```python
from build123d import *

# Parameters (mm, degrees)
SKETCH_1_W      = 10
SKETCH_1_H      = 30
SKETCH_1_R      = 1.5
EXTRUDE_1_DEPTH = 2
FILLET_1_R      = 1


with BuildPart() as part:
    # 草图1 → 凸台-拉伸1 (new body)
    with BuildSketch(Plane.XY):
        with Locations((1.642083631, -16.90903272)):
            Rectangle(SKETCH_1_W, SKETCH_1_H)
        with Locations((1.642083631, -6.90903272)):
            Circle(SKETCH_1_R, mode=Mode.SUBTRACT)
        with Locations((1.642083631, -16.90903272)):
            Circle(SKETCH_1_R, mode=Mode.SUBTRACT)
        with Locations((1.642083631, -26.90903272)):
            Circle(SKETCH_1_R, mode=Mode.SUBTRACT)
    extrude(amount=EXTRUDE_1_DEPTH)

    # 圆角1
    fillet_1_edges = [part.edges().sort_by_distance(p)[0] for p in [
        (-3.357916369, -1.90903272, 1),
        (6.642083631, -1.90903272, 1),
        (6.642083631, -31.90903272, 1),
        (-3.357916369, -31.90903272, 1),
    ]]
    fillet(fillet_1_edges, radius=FILLET_1_R)


solid = part.part
```
Verification items for the finished model (mm, model axes). Give positions to 0.01 mm unless a question says otherwise; leave off trailing zeros. Order: outer loops, then holes, each group sorted by start corner. A loop starts at its lowest first (then second) coordinate and runs counter-clockwise, first axis right, second up. Notation, with made-up numbers: (3, 1.5) - (25, 1.5) arc R20 ccw to (25, 18.5) - close; hole circle Ø10 at (3, -17). An arc over 180 degrees is marked (long way). Answer as CSV lines item,"result". Start each with the question number.
Item 1: Mould release check, pull along X, two halves, no side actions. Record for faces 1 (the face through (6.341, -31.624, 1.014)), 2 (the face through (-1, -17, 2)), 3 (the face through (2.448, -15.644, 0.986)), 4 (the face through (-3.073, -2.21, 1.014)): released by +X, released by -X, zero draft, split by the parting line, or undercut.
Item 2: Gauge pin test, flat end, axial feed: pin 1 (2.5 mm diameter, centred on x = 1.64, y = -26.91, fed in from -Z). Record the tip position at first contact, or that the pin passes through.
Item 3: Section check B-B, the plane x = 1. Record the boundary of the cut face in (y, z).
Item 4: Section check C-C, the plane z = 1. Record the boundary of the cut face in (x, y).
Item 5: Material ranges on L1, parallel to Y at x = 1.5, z = 0.9; L2, parallel to Y at x = 3, z = 0.85; L3, parallel to Y at x = 6.25, z = 1.35, recorded low to high.
Item 6: Section check D-D, the plane y = -16.25. Record the boundary of the cut face in (x, z).
Item 7: Section check A-A, the plane y = -6. Record the boundary of the cut face in (x, z), plus the area to 3 significant figures.
Filled in:
1,face 1,"released by +X"
1,face 2,"zero draft"
1,face 3,"undercut"
1,face 4,"released by -X"
2,pin 1,"through"
3,outline,"(-31.91, 0) - (-28.26, 0) - (-28.26, 2) - (-31.91, 2) - close; (-25.55, 0) - (-18.26, 0) - (-18.26, 2) - (-25.55, 2) - close; (-15.55, 0) - (-8.26, 0) - (-8.26, 2) - (-15.55, 2) - close; (-5.55, 0) - (-1.91, 0) - (-1.91, 2) - (-5.55, 2) - close"
4,outline,"(-3.36, -30.91) arc R1 ccw to (-2.36, -31.91) - (5.64, -31.91) arc R1 ccw to (6.64, -30.91) - (6.64, -2.91) arc R1 ccw to (5.64, -1.91) - (-2.36, -1.91) arc R1 ccw to (-3.36, -2.91) - close; hole circle Ø3 at (1.64, -26.91); hole circle Ø3 at (1.64, -16.91); hole circle Ø3 at (1.64, -6.91)"
5,L1,"-31.91 to -28.4, -25.42 to -18.4, -15.42 to -8.4, -5.42 to -1.91"
5,L2,"-31.91 to -27.55, -26.27 to -17.55, -16.27 to -7.55, -6.27 to -1.91"
5,L3,"-31.7 to -2.12"
6,outline,"(-3.36, 0) - (0.29, 0) - (0.29, 2) - (-3.36, 2) - close; (2.99, 0) - (6.64, 0) - (6.64, 2) - (2.99, 2) - close"
7,outline,"(-3.36, 0) - (0.45, 0) - (0.45, 2) - (-3.36, 2) - close; (2.84, 0) - (6.64, 0) - (6.64, 2) - (2.84, 2) - close"
7,area,"15.2 mm^2"
